```python
from build123d import *

# Parameters (mm, degrees)
F_01_HEX_AF30_DEPTH = 8


with BuildPart() as part:
    # 草图1 → 01_HEX_AF30 (new body)
    with BuildSketch(Plane(origin=(0, 0, 0), x_dir=(0, 0, -1), z_dir=(1, 0, 0))):
        Polygon((17.3205, 0), (8.66025, 14.999993006), (-8.66025, 14.999993006), (-17.3205, 0), (-8.66025, -14.999993006), (8.66025, -14.999993006), align=None)
    extrude(amount=F_01_HEX_AF30_DEPTH)

    # 草图2 → 02_BODY (revolve)
    with BuildSketch(Plane.XY, mode=Mode.PRIVATE) as f_02_body_sk:
        Polygon((8, 0), (8, 8.5), (13, 8.5), (13, 10), (27, 10), (27, 6.5), (34, 6.5), (34, 0), align=None)
    revolve(f_02_body_sk.sketch.rotate(Axis((3, 0, 0), (1, 0, 0)), 90), axis=Axis((3, 0, 0), (1, 0, 0)))


solid = part.part
```
Input: part model. Units: mm. Frame: model coordinates. A direction names the side the tool comes from. Give positions to 0.01 mm unless a question says otherwise; leave off trailing zeros. Order: outer loops, then holes, each group sorted by start corner. A loop starts at its lowest first (then second) coordinate and runs counter-clockwise, first axis right, second up. Notation, with made-up numbers: (-6.5, -17.5) - (39.5, -17.5) arc R23 ccw to (39.5, -4.5) - close; hole circle Ø10 at (1, -35.75). An arc over 180 degrees is marked (long way). One line per item, written item: value.
1. Reachability of faces 1 (the face through (34, 0, 0)), 2 (the face through (20, 0, -10)), 3 (the face through (13, 7.4, 4.5)) from +Z, -Z, +X, -X, +Y, -Y: full face, straight path, thin tool, end or side. Return the list, or none.
Determined:
face 1: +Z, -Z, +X, +Y, -Y
face 2: +X
face 3: none
2. Cut plane A-A, the plane z = -9.5. Output: boundary loops of the cut face in (x, y), and give its area (3 significant figures).
Determined:
outline: (0, -13.55) - (8, -13.55) - (8, 13.55) - (0, 13.55) - close; (13, -3.12) - (27, -3.12) - (27, 3.12) - (13, 3.12) - close
area: 304 mm2
3. Line query: probe 1 along X at (y, z) = (-11.25, -0.5); probe 2 along X at (y, z) = (2.75, 6.5); probe 3 along Z at (x, y) = (7.5, -4). Output: solid intervals per line, ascending.
Determined:
probe 1: 0 to 8
probe 2: 0 to 27
probe 3: -15.01 to 15.01
4. Pin query (flat end, axial travel): pin 1 Ø12 at (x, y) = (22.5, 7) entering from -Z; pin 2 Ø2 at (y, z) = (11.5, 11) entering from +X; pin 3 Ø10 at (x, z) = (16, 6.5) entering from +Y. Return the tip coordinate at first contact, or that it passes through.
Determined:
pin 1: z = -9.95
pin 2: x = 8
pin 3: y = 9.89
5. Cut plane C-C, the plane y = 3.25. Output: boundary loops of the cut face in (x, z), and give its area (3 significant figures).
Determined:
outline: (0, -15.44) - (8, -15.44) - (8, -7.85) - (13, -7.85) - (13, -9.46) - (27, -9.46) - (27, -5.63) - (34, -5.63) - (34, 5.63) - (27, 5.63) - (27, 9.46) - (13, 9.46) - (13, 7.85) - (8, 7.85) - (8, 15.44) - (0, 15.44) - close
area: 669 mm2
6. Draft query along X for faces 4 (the face through (27, 0, 7)), 5 (the face through (10.535, -8.428, -1.107)), 6 (the face through (4, -15, 0)). Return one class per face: released by +X, released by -X, zero draft, split by the parting line, or undercut.
Determined:
face 4: released by +X
face 5: undercut
face 6: zero draft
7. Cut plane B-B, the plane z = 0. Output: boundary loops of the cut face in (x, y).
Determined:
outline: (0, -15) - (8, -15) - (8, -8.5) - (13, -8.5) - (13, -10) - (27, -10) - (27, -6.5) - (34, -6.5) - (34, 6.5) - (27, 6.5) - (27, 10) - (13, 10) - (13, 8.5) - (8, 8.5) - (8, 15) - (0, 15) - close
8. Cut plane D-D, the plane x = 11. Output: boundary loops of the cut face in (y, z).
Determined:
outline: circle Ø17 at (0, 0)
